```python
from build123d import *

# Parameters (mm, degrees)
SKETCH4_W          = 0.666666667
SKETCH4_H          = 0.666666667
CHAMFER1_SIZE      = 0.195
CHAMFER2_SIZE      = 0.625
CHAMFER3_SIZE      = 0.325
CUT_EXTRUDE1_DEPTH = 2.5


with BuildPart() as part:
    # Sketch3 → Revolve1 (revolve)
    with BuildSketch(Plane(origin=(0, 0, 0), x_dir=(0, 0, -1), z_dir=(1, 0, 0))):
        Polygon((-20, 5), (-15, 5), (-15, 3), (10, 3), (10, 2.5), (20, 2.5), (20, 0), (-20, 0), align=None)
    revolve(axis=Axis((0, 0, -20), (0, 0, 1)))

    # Sketch4 → Cut-Revolve1 (revolve, cut)
    with BuildSketch(Plane(origin=(0, 0, 0), x_dir=(0, 0, -1), z_dir=(1, 0, 0))):
        with Locations((-14.666666667, 2.666666667)):
            Rectangle(SKETCH4_W, SKETCH4_H)
    revolve(axis=Axis((0, 0, -20), (0, 0, 1)), mode=Mode.SUBTRACT)

    # Chamfer1
    chamfer1_edges = [part.edges().sort_by_distance(p)[0] for p in [
        (0, -2.333333333, 14.333333333),
        (0, -3, 14.333333333),
    ]]
    chamfer(chamfer1_edges, length=CHAMFER1_SIZE)

    # Sketch6 → Cut-Revolve2 (revolve, cut)
    with BuildSketch(Plane(origin=(0, 0, 0), x_dir=(0, 0, -1), z_dir=(1, 0, 0))):
        with BuildLine():
            Line((10, 3), (13.56, 3))
            Line((13.56, 3), (12.4, 1.84))
            Line((12.4, 1.84), (10.66, 1.84))
            ThreePointArc((10.66, 1.84), (10.193309524, 2.033309524), (10, 2.5))
            Line((10, 2.5), (10, 3))
        make_face()
    revolve(axis=Axis((0, 0, -20), (0, 0, 1)), mode=Mode.SUBTRACT)

    # Chamfer2
    chamfer2_edges = [part.edges().sort_by_distance(p)[0] for p in [
        (0, -2.5, -20),
    ]]
    chamfer(chamfer2_edges, length=CHAMFER2_SIZE)

    # Chamfer3
    chamfer3_edges = [part.edges().sort_by_distance(p)[0] for p in [
        (0, -3, -10),
        (0, -5, 20),
    ]]
    chamfer(chamfer3_edges, length=CHAMFER3_SIZE)

    # Sketch8 → Cut-Extrude1 (cut)
    with BuildSketch(Plane.XY.offset(20)):
        Polygon((1.5, 0.866025404), (0, 1.732050808), (-1.5, 0.866025404), (-1.5, -0.866025404), (0, -1.732050808), (1.5, -0.866025404), align=None)
    extrude(amount=-CUT_EXTRUDE1_DEPTH, mode=Mode.SUBTRACT)


solid = part.part
```
The listing builds one solid part. Answer for the finished solid, in the listing's coordinates (mm). A direction names the side the tool comes from. Give positions to 0.01 mm unless a question says otherwise; leave off trailing zeros. Write each loop counter-clockwise with the first axis right and the second up, starting at its lowest first coordinate (ties: lowest second). Pieces come first, ordered by that corner, then holes. Notation, with made-up numbers: (35.25, -7) - (71.25, -7) arc R19 ccw to (71.25, 13) - close; hole circle Ø5 at (86, 78). An arc over 180 degrees is marked (long way). Use one line per item in the form item = value. Start each with the question number.
1) Consider line 1 along Z through (x, y) = (3.75, 1); line 2 along Z through (x, y) = (2, -2); line 3 along X through (y, z) = (0, 14). Determine where each line is inside the solid, lowest interval first. Write a range as from..to.
2) The mould has two halves that part along X. Classify faces 1 (the face through (0.76, 1.293, 18.768)), 2 (the face through (1.5, 0, 19)), 3 (the face through (-1.824, -0.24, -11.518)), 4 (the face through (0, -2, 20)): pulls with the +X half, pulls with the -X half, needs draft (parallel to the pull), parting line crosses it, or undercut.
3) A tool of negligible diameter and unlimited length cuts with its end or side. For faces 5 (the face through (0, -3, 2)), 6 (the face through (0, 0, -20)), 7 (the face through (0, 0, 17.5)), from which of +Z, -Z, +X, -X, +Y, -Y can it reach the whole face along a straight path? Write none if from no direction.
4) Flat-ended cylindrical pins translate along their axes: pin 1 Ø1.5 at (y, z) = (2, -12) entering from -X; pin 2 Ø2 at (y, z) = (1, 9) entering from -X; pin 3 Ø3 at (y, z) = (0.5, 3.5) entering from +X. Find the tip coordinate at first contact, or state that the pin passes through.
5) Find section A-A on z = 13. Determine the outline of the cut face in (x, y), plus the area to 3 significant figures.
Geometry results:
q1.line_1 = 15..20
q1.line_2 = -9.85..14.31, 15..20
q1.line_3 = -3..3
q2.face_1 = undercut
q2.face_2 = undercut
q2.face_3 = parting line crosses it
q2.face_4 = needs draft
q3.face_5 = -Z
q3.face_6 = -Z, +X, -X, +Y, -Y
q3.face_7 = +Z
q4.pin_1 = -1.35
q4.pin_2 = -3
q4.pin_3 = 3
q5.outline = circle Ø6 at (0, 0)
q5.area = 28.3 mm2
